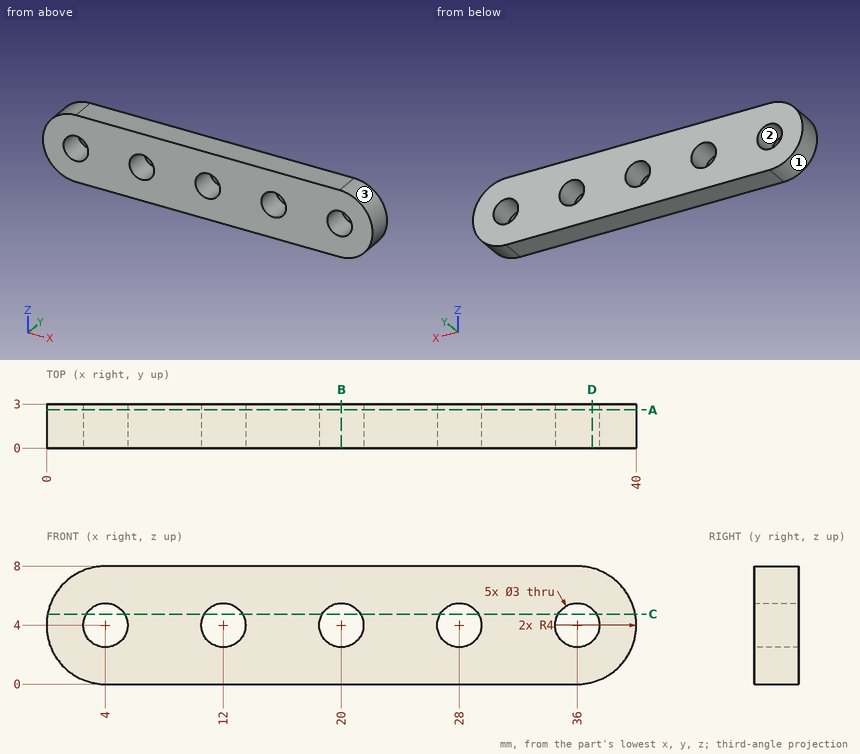
Geometry: see drawing. Coordinates: mm, zero at the bounding-box minimum. Round coordinates to 2 decimals unless told otherwise and drop trailing zeros. Loops run counter-clockwise (first coordinate to the right, second up) from the corner with the lowest first, then second, coordinate; pieces in that order, holes last. Notation, with made-up numbers: M 34,53 L 57,53 A13 cw 57,76 Z; hole C -29.5,2.25 d10. An arc over 180 degrees is marked long. Use a Markdown table: item, result. Add a question column.
1. Mould query, pull axis X, two halves, no side actions, for the marked faces 1, 2 and 3. Classes: pulls with the +X half, pulls with the -X half, needs draft (parallel to the pull), parting line crosses it, or undercut.
2. Section query A-A on y = 2.6. Return the cut outline in (x, z), then the cut area to 3 significant figures.
3. Section query C-C on z = 4.75. Return the cut outline in (x, y), then the cut area to 3 significant figures.
4. Section query D-D on x = 37. Return the cut outline in (y, z).
5. Contact query for a flat-ended pin moving along its axis: P1, Ø2.5, axis at x = 28, z = 4, coming from the -Y side. Output: stop coordinate, or through.
6. Line query: line 1 (X direction, y = 1.2, z = 4); line 2 (X direction, y = 2.7, z = 4.5); line 3 (Z direction, x = 19, y = 1.2). Output: solid intervals per line, ascending.
7. Section query B-B on x = 20. Return the cut outline in (y, z), then the cut area to 3 significant figures.
Reported:
| question | item | result |
|---|---|---|
| 1 | face 1 | pulls with the -X half |
| 1 | face 2 | undercut |
| 1 | face 3 | pulls with the +X half |
| 2 | outline | M 4,0 L 36,0 A4 ccw 36,8 L 4,8 A4 ccw Z; hole C 4,4 d3; hole C 12,4 d3; hole C 20,4 d3; hole C 28,4 d3; hole C 36,4 d3 |
| 2 | area | 271 mm² |
| 3 | outline | M 0.07,0 L 2.7,0 L 2.7,3 L 0.07,3 Z; M 5.3,0 L 10.7,0 L 10.7,3 L 5.3,3 Z; M 13.3,0 L 18.7,0 L 18.7,3 L 13.3,3 Z; M 21.3,0 L 26.7,0 L 26.7,3 L 21.3,3 Z; M 29.3,0 L 34.7,0 L 34.7,3 L 29.3,3 Z; M 37.3,0 L 39.93,0 L 39.93,3 L 37.3,3 Z |
| 3 | area | 80.6 mm² |
| 4 | outline | M 0,0.13 L 3,0.13 L 3,2.88 L 0,2.88 Z; M 0,5.12 L 3,5.12 L 3,7.87 L 0,7.87 Z |
| 5 | P1 | passes through |
| 6 | line 1 | x = 0 to 2.5, 5.5 to 10.5, 13.5 to 18.5, 21.5 to 26.5, 29.5 to 34.5, 37.5 to 40 |
| 6 | line 2 | x = 0.03 to 2.59, 5.41 to 10.59, 13.41 to 18.59, 21.41 to 26.59, 29.41 to 34.59, 37.41 to 39.97 |
| 6 | line 3 | z = 0 to 2.88, 5.12 to 8 |
| 7 | outline | M 0,0 L 3,0 L 3,2.5 L 0,2.5 Z; M 0,5.5 L 3,5.5 L 3,8 L 0,8 Z |
| 7 | area | 15.0 mm² |
